from build123d import *

# Parameters (mm, degrees)
F0_W     = 74.456050992
F0_H     = 65.7130181789
F0_H_2   = 74.0327015519
F1_DEPTH = 60.198
F3_DEPTH = 92.202


with BuildPart() as f1:
    # F0 (on Top) → F1 (new body)
    with BuildSketch(Plane.XY):
        with Locations((37.228025496, -38.9802902937)):
            Rectangle(F0_W, F0_H)
        with Locations((37.228025496, 37.016350776)):
            Rectangle(F0_W, F0_H_2)
        Polygon((-75.2415657043, 0), (0, 0), (0, 74.0327015519), (0, 75.8170485497), (-75.2415657043, 75.8170485497), align=None)
        Polygon((0, -6.1237812042), (0, 0), (-75.2415657043, 0), (-76.6809433699, 0), (-76.6809433699, -71.8367993832), (0, -71.8367993832), align=None)
    extrude(amount=F1_DEPTH)

    # F2 (on Top) → F3 (join)
    with BuildSketch(Plane.XY):
        Polygon((-5.7511497289, 62.2206833214), (-62.2206833214, -5.7511497289), (5.7511497289, -62.2206833214), (62.2206833214, 5.7511497289), align=None)
    extrude(amount=F3_DEPTH)


solid = f1.part
Here's how the part is built. I have some questions about the finished solid (model axes, mm). A direction names the side the tool comes from. Coordinates: 2 decimals unless noted, no trailing zeros. Order: outer loops, then holes, each group sorted by start corner. A loop starts at its lowest first (then second) coordinate and runs counter-clockwise, first axis right, second up. Notation, with made-up numbers: (-3, -18.5) - (17, -18.5) arc R25 cw to (17, -0.5) - close; hole circle Ø7 at (4, 42.5). An arc over 180 degrees is marked (long way). Use CSV: the item, a comma, the result in double quotes. Start each with the question number.
1. I'm going to push flat-ended pins straight in: pin 1 (10 mm diameter, centred on y = 37, z = 19, fed in from -X); pin 2 (24.5 mm diameter, centred on x = 68, z = 30, fed in from +Y); pin 3 (1.5 mm diameter, centred on x = -46.5, y = 47, fed in from +Z). Where does each tip first touch, or does it pass through?
2. Suppose I cut it at A-A on z = 25. List the corners of the cut face in (x, y) for me.
3. Suppose I cut it at B-B on x = 54.5. List the corners of the cut face in (y, z) for me.
4. For faces 1 (the face through (-76.681, -35, 30)), 2 (the face through (-36, 36, 60.198)), 3 (the face through (-33.6, 28.7, 76)), 4 (the face through (37, 74.033, 30)), 5 (the face through (66, 0, 30)), which set-ups out of +Z, -Z, +X, -X, +Y, -Y let a thin tool reach every point of the face, with its end or its side?
5. Suppose I cut it at D-D on x = -53. List the corners of the cut face in (y, z) for me, then the cut area to 3 significant figures.
6. If we mould it in two halves opening along Y, with no side actions, what happens to faces 6 (the face through (-75.242, 38, 30)), 7 (the face through (28.7, 33.6, 76)), 8 (the face through (-28.7, -33.6, 76)), 9 (the face through (63, -6.124, 30))? For each: +Y half, -Y half, draft (parallel to the pull), parting line (faces both ways), or undercut.
7. Suppose I cut it at C-C on y = -30.5. List the corners of the cut face in (x, z) for me.
8. Please list where these lines run through material, in increasing order: line 1 (X direction, y = 37, z = 26); line 2 (Z direction, x = 57, y = 54.5); line 3 (Y direction, x = 17, z = 17). Write a range as from..to.
Output:
1,pin 1,"stops at x = -75.24"
1,pin 2,"stops at y = 74.03"
1,pin 3,"stops at z = 60.2"
2,outline,"(-76.68, -71.84) - (74.46, -71.84) - (74.46, -6.12) - (52.36, -6.12) - (57.44, 0) - (74.46, 0) - (74.46, 74.03) - (0, 74.03) - (0, 75.82) - (-75.24, 75.82) - (-75.24, 0) - (-76.68, 0) - close"
3,outline,"(-71.84, 0) - (-6.12, 0) - (-6.12, 60.2) - (-71.84, 60.2) - close; (-3.54, 0) - (74.03, 0) - (74.03, 60.2) - (12.17, 60.2) - (12.17, 92.2) - (-3.54, 92.2) - close"
4,face 1,"+Z, -Z, -X, +Y, -Y"
4,face 2,"+Z"
4,face 3,"+Z, -X, +Y"
4,face 4,"+Z, -Z, +X, +Y"
4,face 5,"+Z, -Z, +X"
5,outline,"(-71.84, 0) - (75.82, 0) - (75.82, 60.2) - (5.35, 60.2) - (5.35, 92.2) - (-13.41, 92.2) - (-13.41, 60.2) - (-71.84, 60.2) - close"
5,area,"9,490 mm2"
6,face 6,"draft"
6,face 7,"+Y half"
6,face 8,"-Y half"
6,face 9,"undercut"
7,outline,"(-76.68, 0) - (74.46, 0) - (74.46, 60.2) - (32.1, 60.2) - (32.1, 92.2) - (-32.43, 92.2) - (-32.43, 60.2) - (-76.68, 60.2) - close"
8,line 1,"x = -75.24..74.46"
8,line 2,"z = 0..60.2"
8,line 3,"y = -71.84..74.03"
